Autodesk Inventor part; units mm, degrees
ref_plane "YZ Plane" through (0, 0, 0) normal (1, 0, 0) x (0, 1, 0)
ref_plane "XZ Plane" through (0, 0, 0) normal (0, 1, 0) x (-1, 0, 0)
ref_plane "XY Plane" through (0, 0, 0) normal (0, 0, 1) x (1, 0, 0)
sketch "スケッチ1" plane through (0, 0, 0) normal (0, 0, 1) x (1, 0, 0)
  line L0 (0, 0) -> (100, 0)
  line L1 (100, 0) -> (100, 100)
  line L2 (100, 100) -> (0, 100)
  line L3 (0, 100) -> (0, 0)
  dimension "d0" = 100
  dimension "d1" = 100
extrude "押し出し1" add sketch "スケッチ1" along normal blind 5
sketch "スケッチ2" plane through (0, 0, 0) normal (0, -1, 0) x (1, 0, 0)
  line L0 (100, 5) -> (0, 5)
  line L1 (50, 5) -> (50, 0) construction
  line L2 (100, 0) -> (0, 0)
  line L3 (85, 0) -> (15, 0)
  line L4 (15, 0) -> (15, 2.5)
  line L5 (15, 2.5) -> (85, 2.5)
  line L6 (85, 2.5) -> (85, 0)
  point P0 (15, 0)
  dimension "d4" = 70
  dimension "d5" = 2.5
extrude "押し出し2" add sketch "スケッチ2" along normal blind 10
sketch "スケッチ3" plane through (0, 0, 5) normal (0, 0, 1) x (1, 0, 0)
  line L0 (100, 100) -> (0, 100)
  line L1 (50, 100) -> (50, 0) construction
  line L2 (15, 0) -> (85, 0)
  point P0 (0, 0)
  point P1 (50, 20)
  dimension "d15" = 20
hole "穴1" at (50, 20, 5) direction (0, 0, -1) diameter 7 end through all
sketch "スケッチ4" plane through (0, 0, 5) normal (0, 0, 1) x (1, 0, 0)
  line L0 (0, 100) -> (0, 0)
  line L1 (0, 12) -> (100, 12) construction
  line L2 (100, 0) -> (100, 100)
  circle A0 centre (50, 20) radius 3.5
  point P0 (18.5, 12)
  dimension "d16" = 12
  dimension "d17" = 32.5
hole "穴2" at (18.5, 12, 5) direction (0, 0, -1) diameter 22 end through all
sketch "スケッチ5" plane through (0, 100, 0) normal (0, 1, 0) x (1, 0, 0)
  line L0 (15, 0) -> (85, 0)
  line L1 (50, 0) -> (50, -5) construction
  line L2 (53.5, -5) -> (46.5, -5)
  line L3 (15, 0) -> (85, 0)
  line L4 (85, 0) -> (85, -2.5)
  line L5 (85, -2.5) -> (15, -2.5)
  line L6 (15, -2.5) -> (15, 0)
  point P0 (0, 0)
  dimension "d25" = 2.5
  dimension "d26" = 70
extrude "押し出し3" add sketch "スケッチ5" along normal blind 2
properties part number "body_left"
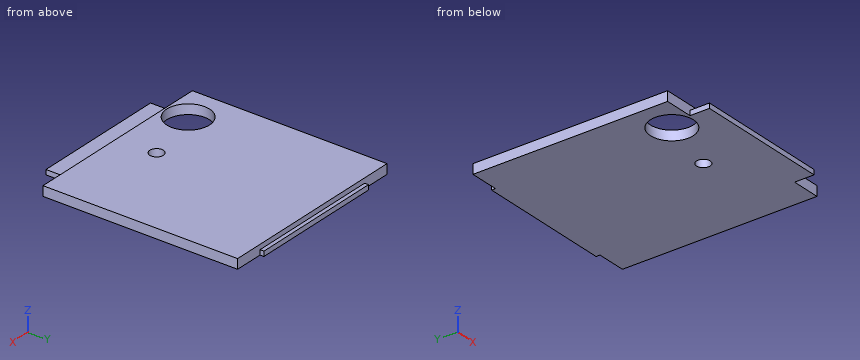
Could you check a few things on this model? Use its own coordinates, in mm. Give positions to 0.01 mm unless a question says otherwise; leave off trailing zeros. Write each loop counter-clockwise with the first axis right and the second up, starting at its lowest first coordinate (ties: lowest second). Pieces come first, ordered by that corner, then holes. Notation, with made-up numbers: (53, 80.5) - (110, 80.5) arc R23 ccw to (110, 104.5) - close; hole circle Ø3 at (45.25, 32). An arc over 180 degrees is marked (long way). One line per item, written item: value. Start each with the question number.
Item 1: Please list where these lines run through material, in increasing order: line 1 (X direction, y = 12, z = 2.85); line 2 (Y direction, x = 18.5, z = 1.6); line 3 (X direction, y = 20, z = 3.2). Write a range as from..to.
Item 2: Imagine slicing it at C-C, the plane z = 1.3. List the corners of the cut face in (x, y) for me, and give its area (3 significant figures).
Item 3: Imagine slicing it at D-D, the plane x = 18.5. List the corners of the cut face in (y, z) for me, and give its area (3 significant figures).
Item 4: Imagine slicing it at A-A, the plane x = 50. List the corners of the cut face in (y, z) for me.
Item 5: I'm going to push flat-ended pins straight in: pin 1 (1 mm diameter, centred on x = 67, y = 101, fed in from +Z); pin 2 (4 mm diameter, centred on x = 50, y = 20, fed in from -Z); pin 3 (1 mm diameter, centred on y = 101, z = 0.5, fed in from -X); pin 4 (1 mm diameter, centred on y = 101, z = 1.5, fed in from +X). Where does each tip first touch, or does it pass through?
Item 6: Imagine slicing it at B-B, the plane y = 12. List the corners of the cut face in (x, z) for me.
Geometry says:
1. line 1: 0..7.5, 29.5..100
1. line 2: -10..1, 23..102
1. line 3: 0..10.95, 26.05..46.5, 53.5..100
2. outline: (0, 0) - (15, 0) - (15, -10) - (85, -10) - (85, 0) - (100, 0) - (100, 100) - (85, 100) - (85, 102) - (15, 102) - (15, 100) - (0, 100) - close; hole circle Ø22 at (18.5, 12); hole circle Ø7 at (50, 20)
2. area: 10,400 mm^2
3. outline: (-10, 0) - (1, 0) - (1, 5) - (0, 5) - (0, 2.5) - (-10, 2.5) - close; (23, 0) - (102, 0) - (102, 2.5) - (100, 2.5) - (100, 5) - (23, 5) - close
3. area: 420 mm^2
4. outline: (-10, 0) - (16.5, 0) - (16.5, 5) - (0, 5) - (0, 2.5) - (-10, 2.5) - close; (23.5, 0) - (102, 0) - (102, 2.5) - (100, 2.5) - (100, 5) - (23.5, 5) - close
5. pin 1: z = 2.5
5. pin 2: through
5. pin 3: x = 15
5. pin 4: x = 85
6. outline: (0, 0) - (7.5, 0) - (7.5, 5) - (0, 5) - close; (29.5, 0) - (100, 0) - (100, 5) - (29.5, 5) - close
